Read the model definition and answer for the solid it produces. Units are mm, in the model's axes. A direction names the side the tool comes from. Round coordinates to 2 decimals unless told otherwise and drop trailing zeros. Order: outer loops, then holes, each group sorted by start corner. A loop starts at its lowest first (then second) coordinate and runs counter-clockwise, first axis right, second up. Notation, with made-up numbers: (-35.75, 53.5) - (-9.75, 53.5) arc R25 ccw to (-9.75, 87.5) - close; hole circle Ø1 at (-17, -36.5). An arc over 180 degrees is marked (long way). Answer as a JSON object with one key per item and string values. Group by question number.
Q1. The mould has two halves that part along X. Classify faces 1 (the flat face through (2, 2, 36)), 2 (the flat face through (-12.5, 0, 17)), 3 (the flat face through (0, -5, 37.2)): pulls with the +X half, pulls with the -X half, needs draft (parallel to the pull), parting line crosses it, or undercut.
Q2. Consider line 1 (Y direction, x = 0, z = 36.55); line 2 (Z direction, x = -4, y = 1.5); line 3 (Z direction, x = 3.5, y = 1.5). Determine where each line is inside the solid, lowest interval first.
Q3. A cutting plane is placed at D-D on x = 5.25. Determine the outline of the cut face in (y, z).
Q4. Given pin 1 Ø5 at (x, z) = (9, 39) entering from +Y; pin 2 Ø4 at (x, z) = (-9.5, 37.5) entering from +Y; pin 3 Ø5 at (x, y) = (0, 9) entering from +Z, each flat-ended and moving along its own axis, determine where each tip first touches the part or whether it passes through.
Q5. A cutting plane is placed at B-B on y = 0. Determine the outline of the cut face in (x, z).
Q6. A tool of negligible diameter and unlimited length cuts with its end or side. For faces 4 (the flat face through (-11.3, 0.2, 35)), 5 (the flat face through (-11.2, -11.3, 17.3)), from which of +Z, -Z, +X, -X, +Y, -Y can it reach the whole face along a straight path? Write none if from no direction.
Q7. A cutting plane is placed at A-A on z = 8.5. Determine the outline of the cut face in (x, y), and give its area (4 significant figures).
```python
from build123d import *

# Parameters (mm, degrees)
SKETCH1_W           = 25
SKETCH1_H           = 25
BOSS_EXTRUDE1_DEPTH = 35
SKETCH2_R           = 11
BOSS_EXTRUDE2_DEPTH = 2.2
CHAMFER1_SIZE       = 2.5
SKETCH4_R           = 4
CUT_EXTRUDE1_DEPTH  = 1.2
SKETCH3_R           = 2.5
BOSS_EXTRUDE3_DEPTH = 20.7


with BuildPart() as part:
    # Sketch1 → Boss-Extrude1 (new body)
    with BuildSketch(Plane.XY):
        Rectangle(SKETCH1_W, SKETCH1_H)
    extrude(amount=BOSS_EXTRUDE1_DEPTH)

    # Sketch2 → Boss-Extrude2 (add)
    with BuildSketch(Plane.XY.offset(35)):
        Circle(SKETCH2_R)
    extrude(amount=BOSS_EXTRUDE2_DEPTH)

    # Chamfer1
    chamfer1_edges = [part.edges().sort_by_distance(p)[0] for p in [
        (12.5, -12.5, 17.5),
        (-12.5, -12.5, 17.5),
        (-12.5, 12.5, 17.5),
        (12.5, 12.5, 17.5),
    ]]
    chamfer(chamfer1_edges, length=CHAMFER1_SIZE)

    # Sketch4 → Cut-Extrude1 (cut)
    with BuildSketch(Plane.XY.offset(37.2)):
        Circle(SKETCH4_R)
    extrude(amount=-CUT_EXTRUDE1_DEPTH, mode=Mode.SUBTRACT)

    # Sketch3 → Boss-Extrude3 (add)
    with BuildSketch(Plane.XY.offset(36)):
        Circle(SKETCH3_R)
    extrude(amount=BOSS_EXTRUDE3_DEPTH)


solid = part.part
```
Result set:
{
 "1": {"face 1": "undercut", "face 2": "pulls with the -X half", "face 3": "needs draft"},
 "2": {"line 1": "y = -11 to -4, -2.5 to 2.5, 4 to 11", "line 2": "z = 0 to 37.2", "line 3": "z = 0 to 36"},
 "3": {"outline": "(-12.5, 0) - (12.5, 0) - (12.5, 35) - (9.67, 35) - (9.67, 37.2) - (-9.67, 37.2) - (-9.67, 35) - (-12.5, 35) - close"},
 "4": {"pin 1": "stops at y = 8.26", "pin 2": "stops at y = 8.03", "pin 3": "stops at z = 37.2"},
 "5": {"outline": "(-12.5, 0) - (12.5, 0) - (12.5, 35) - (11, 35) - (11, 37.2) - (4, 37.2) - (4, 36) - (2.5, 36) - (2.5, 56.7) - (-2.5, 56.7) - (-2.5, 36) - (-4, 36) - (-4, 37.2) - (-11, 37.2) - (-11, 35) - (-12.5, 35) - close"},
 "6": {"face 4": "+Z", "face 5": "+Z, -Z, -X, -Y"},
 "7": {"outline": "(-12.5, -10) - (-10, -12.5) - (10, -12.5) - (12.5, -10) - (12.5, 10) - (10, 12.5) - (-10, 12.5) - (-12.5, 10) - close", "area": "612.5 mm²"}
}
